```python
from build123d import *

# Parameters (mm, degrees)
Y_KSEKLIK_EKSTR_ZYON1_DEPTH      = 10
KES_EKSTR_ZYON1_DEPTH            = 159.748228337
KES_EKSTR_ZYON1_DEPTH_BACK       = 159.748228337
IZIM3_W                          = 1
IZIM3_H                          = 61
PAH1_SIZE                        = 1
Y_KSEKLIK_EKSTR_ZYON2_DEPTH      = 51
Y_KSEKLIK_EKSTR_ZYON2_DEPTH_BACK = 51
IZIM4_W                          = 32
IZIM4_H                          = 89
KES_EKSTR_ZYON2_DEPTH            = 162.632298752
IZIM8_W                          = 32
IZIM8_H                          = 89
KES_EKSTR_ZYON3_DEPTH            = 33.5
KES_EKSTR_ZYON4_DEPTH            = 164.905460556
KES_EKSTR_ZYON4_DEPTH_BACK       = 164.905460556
IZIM9_R                          = 7
KES_EKSTR_ZYON5_DEPTH            = 164.905460556
KES_EKSTR_ZYON5_DEPTH_BACK       = 164.905460556


with BuildPart() as part:
    # Çizim2 → Yükseklik-Ekstrüzyon1 (new, symmetric)
    with BuildSketch(Plane.XY):
        with BuildLine():
            Line((-51, 12.044127192), (-51, 137.955872808))
            ThreePointArc((-51, 137.955872808), (0, 150), (51, 137.955872808))
            Line((51, 137.955872808), (51, 12.044127192))
            ThreePointArc((51, 12.044127192), (0, 0), (-51, 12.044127192))
        make_face()
    extrude(amount=Y_KSEKLIK_EKSTR_ZYON1_DEPTH, both=True)

    # Çizim3 → Kes-Ekstrüzyon1 (cut, two sides: drawn at the far end of the back side and taken through both)
    with BuildSketch(Plane(origin=(0, 0, 0), x_dir=(0, 0, -1), z_dir=(1, 0, 0)).offset(-KES_EKSTR_ZYON1_DEPTH_BACK)):
        with Locations((9.5, 119.5)):
            Rectangle(IZIM3_W, IZIM3_H)
    extrude(amount=KES_EKSTR_ZYON1_DEPTH + KES_EKSTR_ZYON1_DEPTH_BACK, mode=Mode.SUBTRACT)

    # Pah1
    pah1_edges = [part.edges().sort_by_distance(p)[0] for p in [
        (0, 89, -9),
    ]]
    chamfer(pah1_edges, length=PAH1_SIZE - 0.0001)  # a hair under: the kernel refuses the full size

    # Çizim4 → Yükseklik-Ekstrüzyon2 (add, two sides: drawn at the far end of the back side and taken through both)
    with BuildSketch(Plane(origin=(0, 0, 0), x_dir=(0, 0, -1), z_dir=(1, 0, 0)).offset(-Y_KSEKLIK_EKSTR_ZYON2_DEPTH_BACK)):
        with Locations((26, 44.5)):
            Rectangle(IZIM4_W, IZIM4_H)
    extrude(amount=Y_KSEKLIK_EKSTR_ZYON2_DEPTH + Y_KSEKLIK_EKSTR_ZYON2_DEPTH_BACK)

    # Çizim7 → Kes-Ekstrüzyon2 (cut, through all)
    with BuildSketch(Plane.XY.offset(-10)):
        with BuildLine():
            ThreePointArc((0, 0), (-26.201436028, 3.051882621), (-51, 12.044127192))
            Line((-51, 12.044127192), (-51, 0))
            Line((-51, 0), (0, 0))
        make_face()
        with BuildLine():
            ThreePointArc((51, 12.044127192), (26.201436028, 3.051882621), (0, 0))
            Line((0, 0), (51, 0))
            Line((51, 0), (51, 12.044127192))
        make_face()
    extrude(amount=-KES_EKSTR_ZYON2_DEPTH, mode=Mode.SUBTRACT)

    # Çizim8 → Kes-Ekstrüzyon3 (cut, symmetric)
    with BuildSketch(Plane(origin=(0, 0, 0), x_dir=(0, 0, -1), z_dir=(1, 0, 0))):
        with Locations((26, 44.5)):
            Rectangle(IZIM8_W, IZIM8_H)
    extrude(amount=KES_EKSTR_ZYON3_DEPTH, both=True, mode=Mode.SUBTRACT)

    # Çizim9 → Kes-Ekstrüzyon4 (cut, two sides: drawn at the far end of the back side and taken through both)
    with BuildSketch(Plane(origin=(0, 0, 0), x_dir=(0, 0, -1), z_dir=(1, 0, 0)).offset(-KES_EKSTR_ZYON4_DEPTH_BACK)):
        with Locations((26, 75)):
            Circle(IZIM9_R)
    extrude(amount=KES_EKSTR_ZYON4_DEPTH + KES_EKSTR_ZYON4_DEPTH_BACK, mode=Mode.SUBTRACT)

    # Çizim10 → Kes-Döndür1 (revolve, cut)
    with BuildSketch(Plane(origin=(0, 0, 0), x_dir=(0, 0, -1), z_dir=(1, 0, 0)), mode=Mode.PRIVATE) as kes_d_nd_r1_sk:
        Polygon((-10, 35), (-10, 46), (3, 46), (3, 50), (10, 50), (10, 35), align=None)
    revolve(kes_d_nd_r1_sk.sketch.rotate(Axis((0, 35, 10), (0, 0, -1)), 90), axis=Axis((0, 35, 10), (0, 0, -1)), mode=Mode.SUBTRACT)

    # Çizim11 → Kes-Ekstrüzyon5 (cut, two sides: drawn at the far end of the back side and taken through both)
    with BuildSketch(Plane.XY.offset(-KES_EKSTR_ZYON5_DEPTH_BACK)):
        with BuildLine():
            ThreePointArc((29.436953678, 126.900575396), (0, 131.5), (-29.436953678, 126.900575396))
            ThreePointArc((-29.436953678, 126.900575396), (-34.938930721, 116.212813768), (-24.251169092, 110.710836725))
            ThreePointArc((-24.251169092, 110.710836725), (0, 114.5), (24.251169092, 110.710836725))
            ThreePointArc((24.251169092, 110.710836725), (34.938930721, 116.212813768), (29.436953678, 126.900575396))
        make_face()
    extrude(amount=KES_EKSTR_ZYON5_DEPTH + KES_EKSTR_ZYON5_DEPTH_BACK, mode=Mode.SUBTRACT)


solid = part.part
```
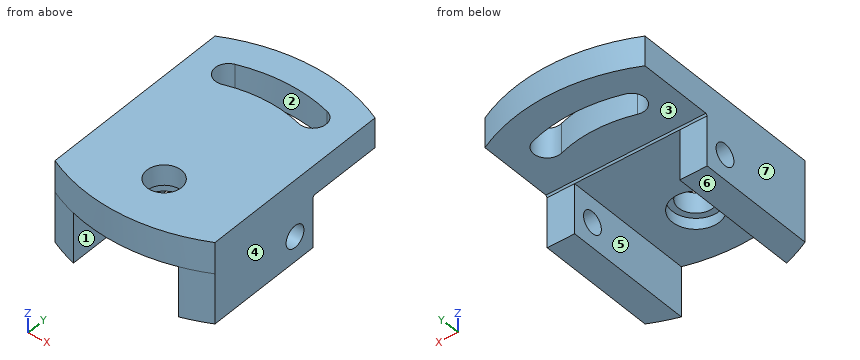
The model under review builds one solid part; all positions refer to its coordinate system, in mm. Face numbers are marked on the shaded views. A direction names the side the tool comes from. Round coordinates to 2 decimals unless told otherwise and drop trailing zeros. Write each loop counter-clockwise with the first axis right and the second up, starting at its lowest first coordinate (ties: lowest second). Pieces come first, ordered by that corner, then holes. Notation, with made-up numbers: (76.5, -33) - (115.5, -33) arc R27 cw to (115.5, -6) - close; hole circle Ø6 at (-24, 3). An arc over 180 degrees is marked (long way). Use one line per item in the form item = value.
Q1. Consider section D-D (x = -21). State the section outline as (y, z) points, and give its area (3 significant figures).
Answer key:
outline = (1.95, -10) - (89, -10) - (90, -9) - (111.68, -9) - (111.68, 10) - (1.95, 10) - close; (129.19, -9) - (148.05, -9) - (148.05, 10) - (129.19, 10) - close
area = 2,530 mm2
Q2. Draft analysis for pull direction X (two halves, no side actions). For the marked faces 4, 5, 6 and 7, state which applies: +X half, -X half, draft (parallel to the pull), parting line (faces both ways), or undercut.
Answer key:
face_4 = +X half
face_5 = undercut
face_6 = draft
face_7 = -X half
Q3. Insertion check: pin 1 Ø8 at (x, z) = (15, -7.5) entering from +Y; pin 2 Ø14 at (x, z) = (46, -19) entering from +Y; pin 3 Ø17.5 at (x, y) = (0, 35) entering from +Z; pin 4 Ø5 at (x, y) = (6.5, 105.5) entering from -Z. Each pin has a flat end and moves straight along its axis. Give the tip position at first contact, or say it passes through.
Answer key:
pin_1 = 149.47
pin_2 = 89
pin_3 = through
pin_4 = -9
Q4. Tool access review of the marked faces 1, 2 and 3: name each direction out of +Z, -Z, +X, -X, +Y, -Y from which nothing blocks a thin tool from reaching the whole face with its end or side.
Answer key:
face_1 = -Z, +Y, -Y
face_2 = +Z, -Z
face_3 = -Z, +X, -X, +Y
Q5. For line 1 (Y direction, x = 0, z = -7.25); line 2 (X direction, y = 24, z = -20.5); line 3 (Z direction, x = -39, y = 75), list the stretches that pass through material, from the lowest coordinate up. Write a range as [from, to].
Answer key:
line_1 = [0, 20], [50, 114.5], [131.5, 150]
line_2 = [-51, -33.5], [33.5, 51]
line_3 = [-42, -33], [-19, 10]
Q6. Consider section A-A (y = 75). State the section outline as (x, z) points.
Answer key:
outline = (-51, -42) - (-33.5, -42) - (-33.5, -33) - (-51, -33) - close; (-51, -19) - (-33.5, -19) - (-33.5, -10) - (33.5, -10) - (33.5, -19) - (51, -19) - (51, 10) - (-51, 10) - close; (33.5, -42) - (51, -42) - (51, -33) - (33.5, -33) - close
Q7. Consider section C-C (z = -38). State the section outline as (x, y) points.
Answer key:
outline = (-51, 12.04) arc R114 ccw to (-33.5, 5.03) - (-33.5, 89) - (-51, 89) - close; (33.5, 5.03) arc R114 ccw to (51, 12.04) - (51, 89) - (33.5, 89) - close
Q8. Consider section B-B (y = 35). State the section outline as (x, z) points, and give its area (3 significant figures).
Answer key:
outline = (-51, -42) - (-33.5, -42) - (-33.5, -10) - (-15, -10) - (-15, -3) - (-11, -3) - (-11, 10) - (-51, 10) - close; (11, -3) - (15, -3) - (15, -10) - (33.5, -10) - (33.5, -42) - (51, -42) - (51, 10) - (11, 10) - close
area = 2,660 mm2
